Geometry check sheet. Reference: the model listing, model coordinates, mm. A direction names the side the tool comes from. Give positions to 0.01 mm unless a question says otherwise; leave off trailing zeros. Write each loop counter-clockwise with the first axis right and the second up, starting at its lowest first coordinate (ties: lowest second). Pieces come first, ordered by that corner, then holes. Notation, with made-up numbers: (19.5, 61) - (67.5, 61) arc R24 cw to (67.5, 96) - close; hole circle Ø5 at (18.5, 30.25). An arc over 180 degrees is marked (long way). Use a Markdown table: item, result.
```python
from build123d import *

# Parameters (mm, degrees)
SKETCH1_W           = 31.8
SKETCH1_H           = 14.75
SKETCH1_R           = 1.5
BOSS_EXTRUDE1_DEPTH = 3


with BuildPart() as part:
    # Sketch1 → Boss-Extrude1 (new body)
    with BuildSketch(Plane.XY):
        with Locations((15.9, 7.375)):
            Rectangle(SKETCH1_W, SKETCH1_H)
        with Locations((29.8, 7.375)):
            Circle(SKETCH1_R, mode=Mode.SUBTRACT)
        with Locations((18.8, 7.375)):
            Circle(SKETCH1_R, mode=Mode.SUBTRACT)
        with Locations((24.3, 12.875)):
            Circle(SKETCH1_R, mode=Mode.SUBTRACT)
        with Locations((24.3, 1.875)):
            Circle(SKETCH1_R, mode=Mode.SUBTRACT)
        with BuildLine():
            Line((5.75, 10.125), (11.25, 10.125))
            ThreePointArc((11.25, 10.125), (14, 7.375), (11.25, 4.625))
            Line((11.25, 4.625), (5.75, 4.625))
            ThreePointArc((5.75, 4.625), (3, 7.375), (5.75, 10.125))
        make_face(mode=Mode.SUBTRACT)
    extrude(amount=BOSS_EXTRUDE1_DEPTH)


solid = part.part
```
1) Material ranges on L1, parallel to Y at x = 24.3, z = 0.85 (3 decimals); L2, parallel to X at y = 7.25, z = 2.5; L3, parallel to Y at x = 29.8, z = 1.8 (3 decimals), recorded low to high. Write a range as from..to.
Working result:
| item | result |
|---|---|
| L1 | y = 0..0.375, 3.375..11.375, 14.375..14.75 |
| L2 | x = 0..3, 14..17.31, 20.29..28.31, 31.29..31.8 |
| L3 | y = 0..5.875, 8.875..14.75 |
2) Section check B-B on x = 29.8. Record the boundary of the cut face in (y, z) (3 decimals), then the cut area to 4 significant figures.
Working result:
| item | result |
|---|---|
| outline | (0, 0) - (5.875, 0) - (5.875, 3) - (0, 3) - close; (8.875, 0) - (14.75, 0) - (14.75, 3) - (8.875, 3) - close |
| area | 35.25 mm² |
3) Section check D-D on z = 1.9. Record the boundary of the cut face in (x, y) (3 decimals), then the cut area to 3 significant figures.
Working result:
| item | result |
|---|---|
| outline | (0, 0) - (31.8, 0) - (31.8, 14.75) - (0, 14.75) - close; hole (5.75, 4.625) - (11.25, 4.625) arc R2.75 ccw to (11.25, 10.125) - (5.75, 10.125) arc R2.75 ccw to start; hole circle Ø3 at (18.8, 7.375); hole circle Ø3 at (24.3, 1.875); hole circle Ø3 at (24.3, 12.875); hole circle Ø3 at (29.8, 7.375) |
| area | 387 mm² |
4) Mould release check, pull along X, two halves, no side actions. Record for faces 3 (the cylindrical face through (25.73, 13.33, 1.48)), 4 (the flat face through (0, 7, 1)), 5 (the flat face through (16, 7, 3)): pulls with the +X half, pulls with the -X half, needs draft (parallel to the pull), parting line crosses it, or undercut.
Working result:
| item | result |
|---|---|
| face 3 | undercut |
| face 4 | pulls with the -X half |
| face 5 | needs draft |
5) Section check A-A on x = 24.3. Record the boundary of the cut face in (y, z) (3 decimals).
Working result:
| item | result |
|---|---|
| outline | (0, 0) - (0.375, 0) - (0.375, 3) - (0, 3) - close; (3.375, 0) - (11.375, 0) - (11.375, 3) - (3.375, 3) - close; (14.375, 0) - (14.75, 0) - (14.75, 3) - (14.375, 3) - close |
6) Set-up check for faces 1 (the flat face through (31.8, 7, 1)), 2 (the cylindrical face through (14, 7.4, 1.5)): record each of +Z, -Z, +X, -X, +Y, -Y from which the full face is reachable in a straight line by a thin tool's end or side.
Working result:
| item | result |
|---|---|
| face 1 | +Z, -Z, +X, +Y, -Y |
| face 2 | +Z, -Z |
7) Section check C-C on y = 13.5. Record the boundary of the cut face in (x, z).
Working result:
| item | result |
|---|---|
| outline | (0, 0) - (22.94, 0) - (22.94, 3) - (0, 3) - close; (25.66, 0) - (31.8, 0) - (31.8, 3) - (25.66, 3) - close |
